Work out the finished part from the listing and answer in its coordinate system (mm). Face numbers are marked on the shaded views. A direction names the side the tool comes from. Coordinates: 2 decimals unless noted, no trailing zeros. Write each loop counter-clockwise with the first axis right and the second up, starting at its lowest first coordinate (ties: lowest second). Pieces come first, ordered by that corner, then holes. Notation, with made-up numbers: (-6.75, 18.25) - (51.25, 18.25) arc R4 ccw to (51.25, 25.25) - close; hole circle Ø9 at (6.25, 55.5). An arc over 180 degrees is marked (long way). Use a Markdown table: item, result. Add a question column.
(1) The part is cut by section D-D, the plane y = -3. Give the vertices of the cut face in (x, z).
(2) The part is cut by section B-B, the plane x = 0. Give the vertices of the cut face in (y, z) (3 decimals).
(3) Find the intervals of material crossed by line 1 (Z direction, x = 6.75, y = -2.75); line 2 (X direction, y = 5.25, z = 2.5); line 3 (Y direction, x = 0, z = 5.25) (3 decimals), in increasing order. Write a range as from..to.
(4) The part is cut by section A-A, the plane z = 4.25. Give the vertices of the cut face in (x, y).
(5) Given pin 1 Ø1 at (y, z) = (2.5, 7.5) entering from +X; pin 2 Ø4 at (y, z) = (5.5, 3) entering from +X; pin 3 Ø3 at (x, z) = (5, 10) entering from +Y, each flat-ended and moving along its own axis, determine where each tip first touches the part or whether it passes through.
(6) For a pull along X with two mould halves and no side action, classify the marked faces 1, 2, 3 and 4 as released by +X, released by -X, zero draft, split by the parting line, or undercut.
(7) The part is cut by section C-C, the plane x = 5. Give the vertices of the cut face in (y, z), then the cut area to 3 significant figures.
(8) A tool of negligible diameter and unlimited length cuts with its end or side. For the marked faces 5, 6 and 7, from which of +Z, -Z, +X, -X, +Y, -Y can it reach the whole face along a straight path? Write none if from no direction.
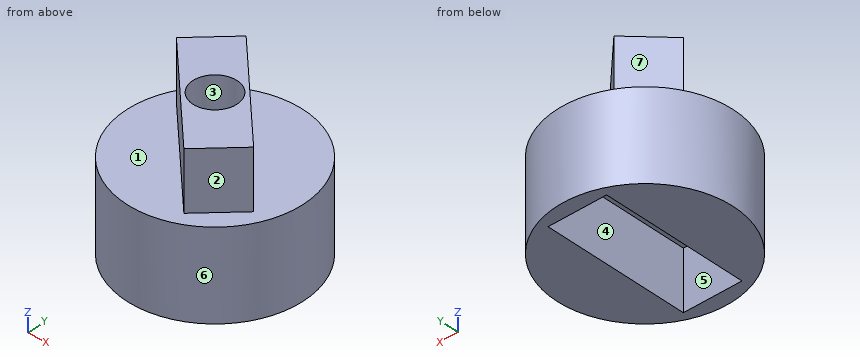
from build123d import *

# Parameters (mm, degrees)
F0_R     = 7.62
F1_DEPTH = 7.62
F2_W     = 5.08
F2_H     = 12.7
F3_DEPTH = 5.08
F5_DEPTH = 5.08
F6_R     = 1.905
F7_DEPTH = 12.701


with BuildPart() as f1:
    # F0 (on Top) → F1 (new body)
    with BuildSketch(Plane.XY):
        Circle(F0_R)
    extrude(amount=F1_DEPTH)

    # F2 (on face) → F3 (cut)
    with BuildSketch(Plane(origin=(0, 0, 0), x_dir=(1, 0, 0), z_dir=(0, 0, -1))):
        Rectangle(F2_W, F2_H)
    extrude(amount=-F3_DEPTH, mode=Mode.SUBTRACT)

    # F4 (on face) → F5 (join)
    with BuildSketch(Plane.XY.offset(7.62)):
        Polygon((-2.694077, 5.837166), (-5.837166, 2.694077), (2.694077, -5.837166), (5.837166, -2.694077), align=None)
    extrude(amount=F5_DEPTH)

    # F6 (on face) → F7 (cut, through all)
    with BuildSketch(Plane.XY.offset(12.7)):
        Circle(F6_R)
    extrude(amount=-F7_DEPTH, mode=Mode.SUBTRACT)


solid = f1.part
Model answer:
| question | item | result |
|---|---|---|
| 1 | outline | (-7, 0) - (-2.54, 0) - (-2.54, 5.08) - (2.54, 5.08) - (2.54, 0) - (7, 0) - (7, 7.62) - (5.53, 7.62) - (5.53, 12.7) - (-0.14, 12.7) - (-0.14, 7.62) - (-7, 7.62) - close |
| 2 | outline | (-7.62, 0) - (-6.35, 0) - (-6.35, 5.08) - (-1.905, 5.08) - (-1.905, 12.7) - (-3.143, 12.7) - (-3.143, 7.62) - (-7.62, 7.62) - close; (1.905, 5.08) - (6.35, 5.08) - (6.35, 0) - (7.62, 0) - (7.62, 7.62) - (3.143, 7.62) - (3.143, 12.7) - (1.905, 12.7) - close |
| 3 | line 1 | 0..7.62 |
| 3 | line 2 | -5.52..-2.54, 2.54..5.52 |
| 3 | line 3 | -7.62..-1.905, 1.905..7.62 |
| 4 | outline | circle Ø15.24 at (0, 0); hole (-2.54, -6.35) - (2.54, -6.35) - (2.54, 6.35) - (-2.54, 6.35) - close |
| 5 | pin 1 | x = 7.35 |
| 5 | pin 2 | x = 6.77 |
| 5 | pin 3 | y = -0.36 |
| 6 | face 1 | zero draft |
| 6 | face 2 | released by +X |
| 6 | face 3 | undercut |
| 6 | face 4 | undercut |
| 7 | outline | (-5.75, 0) - (5.75, 0) - (5.75, 7.62) - (-1.86, 7.62) - (-1.86, 12.7) - (-3.53, 12.7) - (-3.53, 7.62) - (-5.75, 7.62) - close |
| 7 | area | 96.1 mm^2 |
| 8 | face 5 | -Z |
| 8 | face 6 | +Z, -Z |
| 8 | face 7 | +Z, -X, +Y |
